The listing builds one solid part. Answer for the finished solid, in the listing's coordinates (mm). Face numbers are marked on the shaded views. A direction names the side the tool comes from. Give positions to 0.01 mm unless a question says otherwise; leave off trailing zeros. Order: outer loops, then holes, each group sorted by start corner. A loop starts at its lowest first (then second) coordinate and runs counter-clockwise, first axis right, second up. Notation, with made-up numbers: (-33, -14) - (4, -14) arc R17 cw to (4, 2) - close; hole circle Ø6 at (28, -2.75). An arc over 180 degrees is marked (long way). Answer in a Markdown table with one row per item.
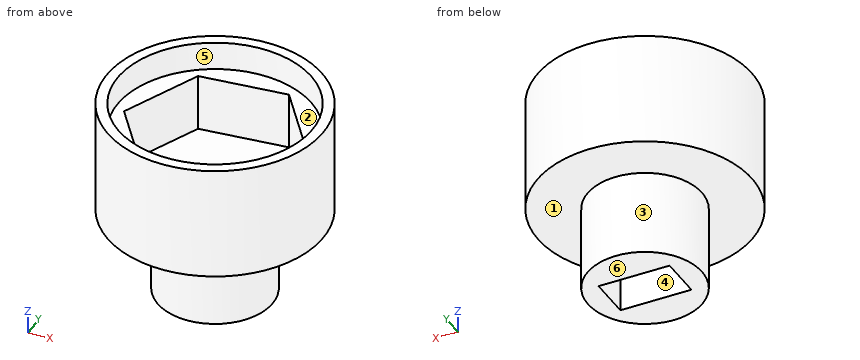
from build123d import *

# Parameters (mm, degrees)
F0_R     = 7.5
F1_DEPTH = 8
F2_R     = 6.75
F3_DEPTH = 2
F5_DEPTH = 4
F6_R     = 4
F7_DEPTH = 6
F8_W     = 5
F8_H     = 3
F9_DEPTH = 6


with BuildPart() as f1:
    # F0 (on Top) → F1 (new body)
    with BuildSketch(Plane.XY):
        Circle(F0_R)
    extrude(amount=F1_DEPTH)

    # F2 (on face) → F3 (cut)
    with BuildSketch(Plane.XY.offset(8)):
        Circle(F2_R)
    extrude(amount=-F3_DEPTH, mode=Mode.SUBTRACT)

    # F4 (on face) → F5 (cut)
    with BuildSketch(Plane.XY.offset(6)):
        Polygon((6.013669, 0.765369), (2.344005, 5.590674), (-3.669664, 4.825305), (-6.013669, -0.765369), (-2.344005, -5.590674), (3.669664, -4.825305), align=None)
    extrude(amount=-F5_DEPTH, mode=Mode.SUBTRACT)

    # F6 (on face) → F7 (join)
    with BuildSketch(Plane(origin=(0, 0, 0), x_dir=(1, 0, 0), z_dir=(0, 0, -1))):
        Circle(F6_R)
    extrude(amount=F7_DEPTH)

    # F8 (on face) → F9 (cut)
    with BuildSketch(Plane(origin=(0, 0, -6), x_dir=(1, 0, 0), z_dir=(0, 0, -1))):
        Rectangle(F8_W, F8_H)
    extrude(amount=-F9_DEPTH, mode=Mode.SUBTRACT)


solid = f1.part
Item 1: Determine the mould class of the marked faces 1, 2 and 3 for opening direction X: pulls with the +X half, pulls with the -X half, needs draft (parallel to the pull), parting line crosses it, or undercut.
Answer block:
| item | result |
|---|---|
| face 1 | needs draft |
| face 2 | undercut |
| face 3 | parting line crosses it |
Item 2: Each of these flat-tipped pins is pushed along its axis until it touches: P1, Ø1, axis at y = 3, z = 2, coming from the +X side; P2, Ø3, axis at x = 3.5, z = 2.5, coming from the +Y side; P3, Ø0.9, axis at y = 0.5, z = -4, coming from the +X side. Where does it stop, or does it pass through?
Answer block:
| item | result |
|---|---|
| P1 | x = 7.07 |
| P2 | y = 7.23 |
| P3 | x = 4 |
Item 3: Find section C-C on y = 4.25. Write down the section's boundary in (x, z), then the cut area to 3 significant figures.
Answer block:
| item | result |
|---|---|
| outline | (-6.18, 0) - (6.18, 0) - (6.18, 8) - (5.24, 8) - (5.24, 6) - (3.36, 6) - (3.36, 2) - (-3.91, 2) - (-3.91, 6) - (-5.24, 6) - (-5.24, 8) - (-6.18, 8) - close |
| area | 48.8 mm² |
Item 4: Find section A-A on z = -1.75. Write down the section's boundary in (x, y).
Answer block:
| item | result |
|---|---|
| outline | circle Ø8 at (0, 0); hole (-2.5, -1.5) - (2.5, -1.5) - (2.5, 1.5) - (-2.5, 1.5) - close |
Item 5: Find section B-B on x = 0. Write down the section's boundary in (y, z), then the cut area to 3 significant figures.
Answer block:
| item | result |
|---|---|
| outline | (-7.5, 0) - (-4, 0) - (-4, -6) - (-1.5, -6) - (-1.5, 0) - (1.5, 0) - (1.5, -6) - (4, -6) - (4, 0) - (7.5, 0) - (7.5, 8) - (6.75, 8) - (6.75, 6) - (5.29, 6) - (5.29, 2) - (-5.29, 2) - (-5.29, 6) - (-6.75, 6) - (-6.75, 8) - (-7.5, 8) - close |
| area | 80.7 mm² |
Item 6: Which of the six approach directions +Z, -Z, +X, -X, +Y, -Y give full straight-line access (tool end or side, diameter ignored) to the marked faces 4, 5 and 6?
Answer block:
| item | result |
|---|---|
| face 4 | -Z |
| face 5 | +Z |
| face 6 | -Z, +X, -X, +Y, -Y |
Item 7: Consider line 1 (Y direction, x = 0, z = 6.85); line 2 (Z direction, x = 5.75, y = -0.25); line 3 (Z direction, x = 1.5, y = -4.75). Determine where each line is inside the solid, lowest interval first.
Answer block:
| item | result |
|---|---|
| line 1 | -7.5 to -6.75, 6.75 to 7.5 |
| line 2 | 0 to 6 |
| line 3 | 0 to 2 |
Item 8: Find section D-D on z = 0.5. Write down the section's boundary in (x, y), then the cut area to 3 significant figures.
Answer block:
| item | result |
|---|---|
| outline | circle Ø15 at (0, 0) |
| area | 177 mm² |
